from build123d import *

# Parameters (mm, degrees)
F1_DEPTH = 1.5875
F2_W     = 15.875
F2_H     = 11.1125
F3_DEPTH = 11.1125
F4_W     = 1.5875
F4_H     = 9.144
F4_W_2   = 12.7
F5_DEPTH = 9.525
F6_W     = 26.9875
F6_H     = 3.175
F6_W_2   = 20.6375
F6_W_3   = 15.875
F7_DEPTH = 9.525


with BuildPart() as f1:
    # F0 (on Top) → F1 (new body)
    with BuildSketch(Plane.XY):
        Polygon((-38.356409, 37.185692), (-38.356409, -13.083157), (28.445591, -13.083157), (28.445591, -11.495657), (31.317557, -10.141982), (31.317557, 23.132018), (28.445591, 24.485692), (28.445591, 37.185692), align=None)
    extrude(amount=F1_DEPTH)

    # F2 (on face) → F3 (join)
    with BuildSketch(Plane.XY.offset(1.5875)):
        with Locations((-36.768909, 22.104442)):
            Rectangle(F2_W, F2_H)
    extrude(amount=F3_DEPTH)

    # F4 (on face) → F5 (join)
    with BuildSketch(Plane.XY.offset(1.5875)):
        with Locations((-39.150159, -5.336157)):
            Rectangle(F4_W, F4_H)
        with Locations((-32.006409, -5.336157)):
            Rectangle(F4_W_2, F4_H)
    extrude(amount=F5_DEPTH)

    # F6 (on face) → F7 (join)
    with BuildSketch(Plane.XY.offset(1.5875)):
        with Locations((-8.066909, 34.010692)):
            Rectangle(F6_W, F6_H)
        with Locations((16.539341, 34.010692)):
            Rectangle(F6_W_2, F6_H)
        with Locations((-0.923159, -9.908157)):
            Rectangle(F6_W_2, F6_H)
        with Locations((18.920591, -9.908157)):
            Rectangle(F6_W_3, F6_H)
    extrude(amount=F7_DEPTH)


solid = f1.part
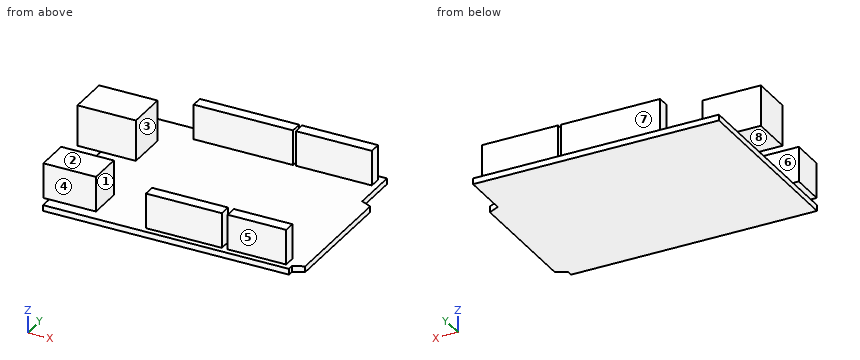
Read the model definition and answer for the solid it produces. Units are mm, in the model's axes. Face numbers are marked on the shaded views. A direction names the side the tool comes from. Give positions to 0.01 mm unless a question says otherwise; leave off trailing zeros. Loops run counter-clockwise (first coordinate to the right, second up) from the corner with the lowest first, then second, coordinate; pieces in that order, holes last. Notation, with made-up numbers: (-10.5, 27) -> (9.5, 27) arc R17 cw to (9.5, 57) -> close; hole circle Ø3 at (56, 57.25). An arc over 180 degrees is marked (long way). Use a Markdown table: item, result.
Q1. Section D-D, the plane y = -4.5 is taken. Determine the outline of the cut face in (x, z), then the cut area to 3 significant figures.
Solved:
| item | result |
|---|---|
| outline | (-39.94, 1.59) -> (-38.36, 1.59) -> (-38.36, 0) -> (31.32, 0) -> (31.32, 1.59) -> (-25.66, 1.59) -> (-25.66, 11.11) -> (-39.94, 11.11) -> close |
| area | 247 mm^2 |
Q2. Section B-B, the plane y = 18.5 is taken. Determine the outline of the cut face in (x, z), then the cut area to 3 significant figures.
Solved:
| item | result |
|---|---|
| outline | (-44.71, 1.59) -> (-38.36, 1.59) -> (-38.36, 0) -> (31.32, 0) -> (31.32, 1.59) -> (-28.83, 1.59) -> (-28.83, 12.7) -> (-44.71, 12.7) -> close |
| area | 287 mm^2 |
Q3. A tool of negligible diameter and unlimited length cuts with its end or side. For the marked faces 4, 5, 6, 7 and 8, from which of +Z, -Z, +X, -X, +Y, -Y can it reach the whole face along a straight path? Write none if from no direction.
Solved:
| item | result |
|---|---|
| face 4 | +Z, -X, -Y |
| face 5 | +Z, +X, -X, -Y |
| face 6 | +Z, +X, -X |
| face 7 | +Z, +X, -X, +Y |
| face 8 | -Z, -X, +Y, -Y |
Q4. Find the intervals of material crossed by line 1 along X through (y, z) = (-8.5, 5); line 2 along Y through (x, z) = (25.5, 3.5); line 3 along X through (y, z) = (33.5, 5.25), in increasing order.
Solved:
| item | result |
|---|---|
| line 1 | x = -39.94 to -25.66, -11.24 to 9.4, 10.98 to 26.86 |
| line 2 | y = -11.5 to -8.32, 32.42 to 35.6 |
| line 3 | x = -21.56 to 5.43, 6.22 to 26.86 |
Q5. Section C-C, the plane x = -3.5 is taken. Determine the outline of the cut face in (y, z), then the cut area to 3 significant figures.
Solved:
| item | result |
|---|---|
| outline | (-13.08, 0) -> (37.19, 0) -> (37.19, 1.59) -> (35.6, 1.59) -> (35.6, 11.11) -> (32.42, 11.11) -> (32.42, 1.59) -> (-8.32, 1.59) -> (-8.32, 11.11) -> (-11.5, 11.11) -> (-11.5, 1.59) -> (-13.08, 1.59) -> close |
| area | 140 mm^2 |
Q6. Section A-A, the plane z = 5.75 is taken. Determine the outline of the cut face in (x, y).
Solved:
| item | result |
|---|---|
| outline | (-44.71, 16.55) -> (-28.83, 16.55) -> (-28.83, 27.66) -> (-44.71, 27.66) -> close; (-39.94, -9.91) -> (-25.66, -9.91) -> (-25.66, -0.76) -> (-39.94, -0.76) -> close; (-21.56, 32.42) -> (5.43, 32.42) -> (5.43, 35.6) -> (-21.56, 35.6) -> close; (-11.24, -11.5) -> (9.4, -11.5) -> (9.4, -8.32) -> (-11.24, -8.32) -> close; (6.22, 32.42) -> (26.86, 32.42) -> (26.86, 35.6) -> (6.22, 35.6) -> close; (10.98, -11.5) -> (26.86, -11.5) -> (26.86, -8.32) -> (10.98, -8.32) -> close |
Q7. Each of these flat-tipped pins is pushed along its axis until it touches: pin 1 (7.5 mm diameter, centred on x = -35.5, y = -5, fed in from +Z); pin 2 (1 mm diameter, centred on y = -10, z = 8, fed in from -X); pin 3 (7.5 mm diameter, centred on x = -35.5, z = 5.5, fed in from -Y). Where does it stop, or does it pass through?
Solved:
| item | result |
|---|---|
| pin 1 | stops at z = 11.11 |
| pin 2 | stops at x = -39.94 |
| pin 3 | stops at y = -9.91 |
Q8. Determine the mould class of the marked faces 1, 2 and 3 for opening direction X: pulls with the +X half, pulls with the -X half, needs draft (parallel to the pull), parting line crosses it, or undercut.
Solved:
| item | result |
|---|---|
| face 1 | undercut |
| face 2 | needs draft |
| face 3 | pulls with the +X half |
